Source: three-view drawing plus pictorial views. Frame: mm from the lowest corner of the part. A direction names the side the tool comes from. Coordinates: 2 decimals unless noted, no trailing zeros. Write each loop counter-clockwise with the first axis right and the second up, starting at its lowest first coordinate (ties: lowest second). Pieces come first, ordered by that corner, then holes. Notation, with made-up numbers: (41.25, 79) -> (55.25, 79) arc R27 ccw to (55.25, 112) -> close; hole circle Ø6 at (7.25, -27). An arc over 180 degrees is marked (long way). One line per item, written item: value.
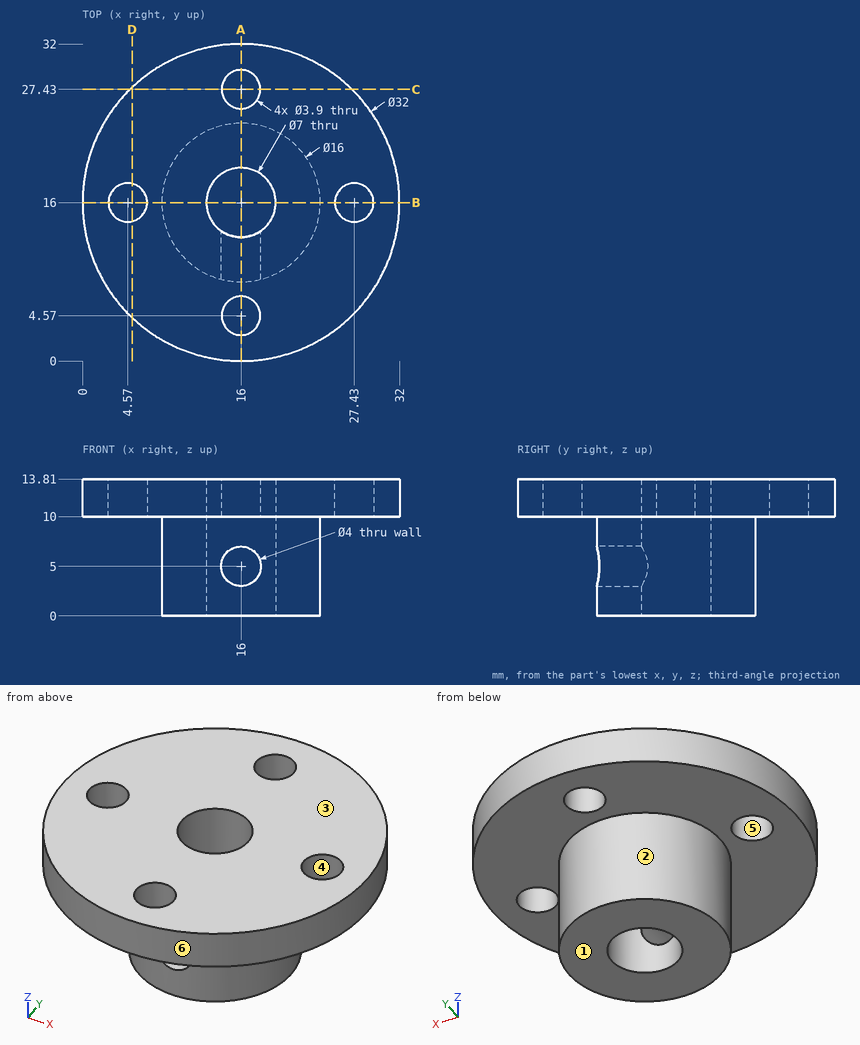
(1) Line query: line 1 (Y direction, x = 16, z = 11.4); line 2 (Z direction, x = 10.5, y = 3.5); line 3 (X direction, y = 10, z = 6). Output: solid intervals per line, ascending. Write a range as [from, to].
Responses:
line 1: y = [0, 2.62], [6.52, 12.5], [19.5, 25.48], [29.38, 32]
line 2: z = [10, 13.81]
line 3: x = [10.71, 14.27], [17.73, 21.29]
(2) Pull-direction query (Y, two-part tool) for the marked faces 3, 4, 5 and 6; classes: released by +Y, released by -Y, zero draft, split by the parting line, or undercut.
Responses:
face 3: zero draft
face 4: undercut
face 5: undercut
face 6: split by the parting line
(3) Section A-A (x = 16). Return the cut outline in (y, z), then the cut area to 3 significant figures.
Responses:
outline: (0, 10) -> (2.62, 10) -> (2.62, 13.81) -> (0, 13.81) -> close; (6.52, 10) -> (8, 10) -> (8, 7) -> (12.5, 7) -> (12.5, 13.81) -> (6.52, 13.81) -> close; (8, 0) -> (12.5, 0) -> (12.5, 3) -> (8, 3) -> close; (19.5, 0) -> (24, 0) -> (24, 10) -> (25.48, 10) -> (25.48, 13.81) -> (19.5, 13.81) -> close; (29.38, 10) -> (32, 10) -> (32, 13.81) -> (29.38, 13.81) -> close
area: 138 mm2
(4) Section D-D (x = 5). Return the cut outline in (y, z), then the cut area to 3 significant figures.
Responses:
outline: (4.38, 10) -> (14.1, 10) -> (14.1, 13.81) -> (4.38, 13.81) -> close; (17.9, 10) -> (27.62, 10) -> (27.62, 13.81) -> (17.9, 13.81) -> close
area: 74.0 mm2
(5) First-contact query: pin 1 (1 mm diameter, centred on y = 11, z = 4, fed in from +X); pin 2 (1.5 mm diameter, centred on x = 8, z = 3, fed in from +Y); pin 3 (5 mm diameter, centred on x = 3.5, y = 19.5, fed in from -Z). Flat tips, straight axial feed; report the tip coordinate or a pass-through.
Responses:
pin 1: stops at x = 22.61
pin 2: stops at y = 19.38
pin 3: stops at z = 10
(6) Section C-C (y = 27.43). Return the cut outline in (x, z), then the cut area to 3 significant figures.
Responses:
outline: (4.8, 10) -> (14.05, 10) -> (14.05, 13.81) -> (4.8, 13.81) -> close; (17.95, 10) -> (27.2, 10) -> (27.2, 13.81) -> (17.95, 13.81) -> close
area: 70.5 mm2
(7) Reachability of the marked faces 1 and 2 from +Z, -Z, +X, -X, +Y, -Y: full face, straight path, thin tool, end or side. Return the list, or none.
Responses:
face 1: -Z, +X, -X, +Y, -Y
face 2: -Z
(8) Section B-B (y = 16). Return the cut outline in (x, z), then the cut area to 3 significant figures.
Responses:
outline: (0, 10) -> (2.62, 10) -> (2.62, 13.81) -> (0, 13.81) -> close; (6.52, 10) -> (8, 10) -> (8, 0) -> (12.5, 0) -> (12.5, 13.81) -> (6.52, 13.81) -> close; (19.5, 0) -> (24, 0) -> (24, 10) -> (25.48, 10) -> (25.48, 13.81) -> (19.5, 13.81) -> close; (29.38, 10) -> (32, 10) -> (32, 13.81) -> (29.38, 13.81) -> close
area: 156 mm2
